Part model, mm, in its own coordinate system. Face numbers are marked on the shaded views. A direction names the side the tool comes from. Coordinates: 2 decimals unless noted, no trailing zeros. Write each loop counter-clockwise with the first axis right and the second up, starting at its lowest first coordinate (ties: lowest second). Pieces come first, ordered by that corner, then holes. Notation, with made-up numbers: (86.25, 87) - (142.25, 87) arc R11 ccw to (142.25, 98) - close; hole circle Ø2 at (-25.75, -23.75). An arc over 180 degrees is marked (long way). Use a Markdown table: item, result.
```python
from build123d import *

# Parameters (mm, degrees)
SKETCH1_R           = 7
BOSS_EXTRUDE1_DEPTH = 4.2
SKETCH2_R           = 3
CUT_EXTRUDE1_DEPTH  = 4.2
SKETCH3_R           = 6.75
SKETCH3_R_2         = 4.5
CUT_EXTRUDE2_DEPTH  = 1.25
SKETCH4_R           = 4
SKETCH4_R_2         = 3
BOSS_EXTRUDE2_DEPTH = 2.8
FILLET1_R           = 0.1


with BuildPart() as part:
    # Sketch1 → Boss-Extrude1 (new body)
    with BuildSketch(Plane(origin=(0, 0, 0), x_dir=(1, 0, 0), z_dir=(0, 1, 0))):
        Circle(SKETCH1_R)
    extrude(amount=BOSS_EXTRUDE1_DEPTH)

    # Sketch2 → Cut-Extrude1 (cut)
    with BuildSketch(Plane(origin=(0, 4.2, 0), x_dir=(1, 0, 0), z_dir=(0, 1, 0))):
        Circle(SKETCH2_R)
    extrude(amount=-CUT_EXTRUDE1_DEPTH, mode=Mode.SUBTRACT)

    # Sketch3 → Cut-Extrude2 (cut)
    with BuildSketch(Plane(origin=(0, 4.2, 0), x_dir=(1, 0, 0), z_dir=(0, 1, 0))):
        Circle(SKETCH3_R)
        Circle(SKETCH3_R_2, mode=Mode.SUBTRACT)
    extrude(amount=-CUT_EXTRUDE2_DEPTH, mode=Mode.SUBTRACT)

    # Sketch4 → Boss-Extrude2 (add)
    with BuildSketch(Plane.XZ):
        Circle(SKETCH4_R)
        Circle(SKETCH4_R_2, mode=Mode.SUBTRACT)
    extrude(amount=BOSS_EXTRUDE2_DEPTH)

    # Fillet1
    fillet1_edges = [part.edges().sort_by_distance(p)[0] for p in [
        (-4, -2.8, 0),
    ]]
    fillet(fillet1_edges, radius=FILLET1_R)


solid = part.part
```
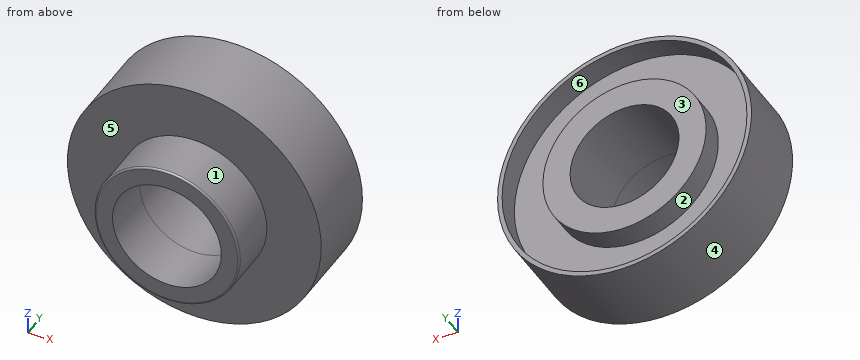
Item 1: Which spindle directions (+Z, -Z, +X, -X, +Y, -Y) get a long thin tool onto all of the face, cutting with end or side? Do the marked faces 1, 2 and 3. Say none if no direction does.
From the geometry:
| item | result |
|---|---|
| face 1 | -Y |
| face 2 | +Y |
| face 3 | +Z, -Z, +X, -X, +Y |
Item 2: Band-saw the part on D-D, the plane x = -5.5. Give the cut face in (y, z).
From the geometry:
| item | result |
|---|---|
| outline | (0, -4.33) - (4.2, -4.33) - (4.2, -3.91) - (2.95, -3.91) - (2.95, 3.91) - (4.2, 3.91) - (4.2, 4.33) - (0, 4.33) - close |
Item 3: Drop flat-ended pins along their axis: P1, Ø3, axis at y = 1.5, z = -3, coming from the -X side; P2, Ø3, axis at x = 0, y = -2, coming from the -Z side. Give the stop position or say it passes through.
From the geometry:
| item | result |
|---|---|
| P1 | x = -6.84 |
| P2 | z = -4 |
Item 4: Drill centre lines: probe 1 along X at (y, z) = (3.1, 0); probe 2 along X at (y, z) = (1.25, 0); probe 3 along Z at (x, y) = (-0.75, 3.5). Where is each one in solid material? Low to high.
From the geometry:
| item | result |
|---|---|
| probe 1 | -7 to -6.75, -4.5 to -3, 3 to 4.5, 6.75 to 7 |
| probe 2 | -7 to -3, 3 to 7 |
| probe 3 | -6.96 to -6.71, -4.44 to -2.9, 2.9 to 4.44, 6.71 to 6.96 |
Item 5: Two-plate mould, pull along Z, no slides. Class the marked faces 4, 5 and 6: pulls with the +Z half, pulls with the -Z half, needs draft (parallel to the pull), parting line crosses it, or undercut.
From the geometry:
| item | result |
|---|---|
| face 4 | parting line crosses it |
| face 5 | needs draft |
| face 6 | undercut |
Item 6: Band-saw the part on B-B, the plane z = 0. Give the cut face in (x, y).
From the geometry:
| item | result |
|---|---|
| outline | (-7, 0) - (-4, 0) - (-4, -2.7) arc R0.1 ccw to (-3.9, -2.8) - (-3, -2.8) - (-3, 4.2) - (-4.5, 4.2) - (-4.5, 2.95) - (-6.75, 2.95) - (-6.75, 4.2) - (-7, 4.2) - close; (3, -2.8) - (3.9, -2.8) arc R0.1 ccw to (4, -2.7) - (4, 0) - (7, 0) - (7, 4.2) - (6.75, 4.2) - (6.75, 2.95) - (4.5, 2.95) - (4.5, 4.2) - (3, 4.2) - close |
Item 7: Band-saw the part on C-C, the plane y = 2.5. Give the cut face in (x, z), then the cut area to 3 significant figures.
From the geometry:
| item | result |
|---|---|
| outline | circle Ø14 at (0, 0); hole circle Ø6 at (0, 0) |
| area | 126 mm^2 |
Item 8: Band-saw the part on A-A, the plane x = 0. Give the cut face in (y, z), then the cut area to 3 significant figures.
From the geometry:
| item | result |
|---|---|
| outline | (-2.8, -3.9) arc R0.1 ccw to (-2.7, -4) - (0, -4) - (0, -7) - (4.2, -7) - (4.2, -6.75) - (2.95, -6.75) - (2.95, -4.5) - (4.2, -4.5) - (4.2, -3) - (-2.8, -3) - close; (-2.8, 3) - (4.2, 3) - (4.2, 4.5) - (2.95, 4.5) - (2.95, 6.75) - (4.2, 6.75) - (4.2, 7) - (0, 7) - (0, 4) - (-2.7, 4) arc R0.1 ccw to (-2.8, 3.9) - close |
| area | 33.6 mm^2 |
